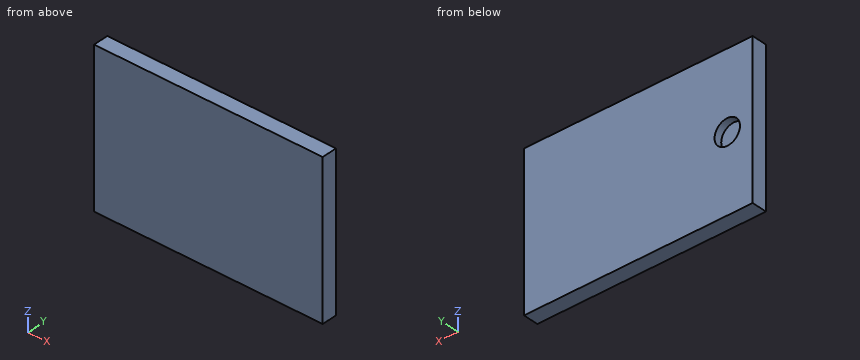
from build123d import *

# Parameters (mm, degrees)
F0_W     = 45
F0_H     = 30
F1_DEPTH = 1.5
F2_D     = 5
F2_DEPTH = 1.501


with BuildPart() as f1:
    # F0 (on Front) → F1 (new body, symmetric)
    with BuildSketch(Plane.XZ):
        with Locations((-9.7826488498, 10.1560708135)):
            Rectangle(F0_W, F0_H)
    extrude(amount=F1_DEPTH, both=True)

    # F2 (through all, one way)
    with BuildSketch(Plane.XZ):
        with Locations((-27.2826488498, 10.1560708135)):
            Circle(F2_D / 2)
    extrude(amount=-F2_DEPTH, mode=Mode.SUBTRACT)


solid = f1.part
CAD build for the part. Positions are in the model's coordinates, mm. Round coordinates to 2 decimals unless told otherwise and drop trailing zeros. Order: outer loops, then holes, each group sorted by start corner. A loop starts at its lowest first (then second) coordinate and runs counter-clockwise, first axis right, second up. Notation, with made-up numbers: M 39,83 L 49,83 A26 ccw 49,100 Z; hole C 20,1 d5. An arc over 180 degrees is marked long. Use one line per item in the form item = value.
Q1. Saw through at A-A on z = 8.5. Give the cut face in (x, y), then the cut area to 3 significant figures.
Recorded:
outline = M -32.28,-1.5 L 12.72,-1.5 L 12.72,1.5 L -25.41,1.5 L -25.41,0 L -29.16,0 L -29.16,1.5 L -32.28,1.5 Z
area = 129 mm^2
Q2. Flat gauge pin, fed straight in: P1, Ø2.5, axis at x = -28, z = 11, coming from the +Y side. Where does the tip first touch, or does it go through?
Recorded:
P1 = 0
Q3. Probe L1, parallel to X at y = 0.35, z = 11.75; L2, parallel to X at y = 0.9, z = 12.25; L3, parallel to Z at x = -25, y = 0.9. List the from-to ranges inside material, lowest first.
Recorded:
L1 = -32.28 to -29.21, -25.36 to 12.72
L2 = -32.28 to -28.65, -25.92 to 12.72
L3 = -4.84 to 9.14, 11.18 to 25.16
